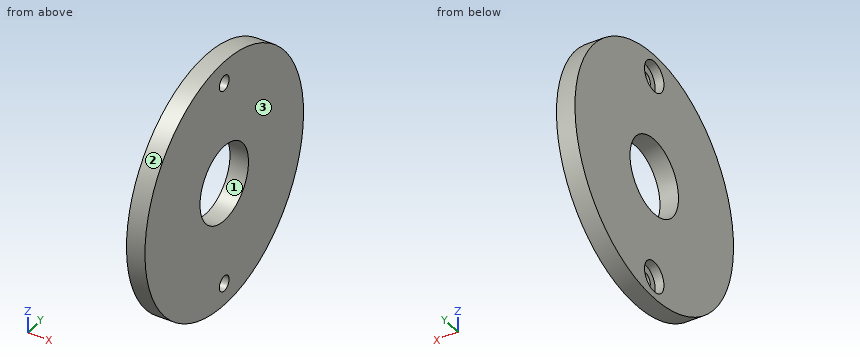
from build123d import *

# Parameters (mm, degrees)
F0_W     = 6.3
F0_H     = 29.5
F2_R     = 2.6
F3_DEPTH = 25
F4_R     = 5.2
F4_R_2   = 2.6
F5_DEPTH = 3


with BuildPart() as f1:
    # F0 (on Front) → F1 (revolve)
    with BuildSketch(Plane.XZ):
        with Locations((5.599999, 27.75)):
            Rectangle(F0_W, F0_H)
    revolve(axis=Axis((-4.686111, 0, 0), (-1, 0, 0)))

    # F2 (on face) → F3 (cut)
    with BuildSketch(Plane(origin=(2.449999, 0, 0), x_dir=(0, -1, 0), z_dir=(-1, 0, 0))):
        with Locations((0, 35)):
            Circle(F2_R)
        with Locations((0, -35)):
            Circle(F2_R)
    extrude(amount=-F3_DEPTH, mode=Mode.SUBTRACT)

    # F4 (on face) → F5 (cut)
    with BuildSketch(Plane(origin=(2.449999, 0, 0), x_dir=(0, -1, 0), z_dir=(-1, 0, 0))):
        with Locations((0, 35)):
            Circle(F4_R)
        with Locations((0, 35)):
            Circle(F4_R_2, mode=Mode.SUBTRACT)
        with Locations((0, -35)):
            Circle(F4_R)
        with Locations((0, -35)):
            Circle(F4_R_2, mode=Mode.SUBTRACT)
    extrude(amount=-F5_DEPTH, mode=Mode.SUBTRACT)


solid = f1.part
Can you work these out from the model? Positions are in its coordinate system, mm. Face numbers are marked on the shaded views. Give positions to 0.01 mm unless a question says otherwise; leave off trailing zeros. Loops run counter-clockwise (first coordinate to the right, second up) from the corner with the lowest first, then second, coordinate; pieces in that order, holes last. Notation, with made-up numbers: (86, -17) - (108, -17) arc R20 ccw to (108, 4) - close; hole circle Ø1 at (-4, -25.75). An arc over 180 degrees is marked (long way). Return JSON: item names as keys, results as strings.
1. I want a section at C-C on x = 3.5. Please give me the cut outline in (y, z).
Output values:
{"outline": "circle Ø85 at (0, 0); hole circle Ø26 at (0, 0); hole circle Ø10.4 at (0, -35); hole circle Ø10.4 at (0, 35)"}
2. We'd pull the mould along Z, two halves only. Please class the marked faces 1, 2 and 3: +Z half, -Z half, draft (parallel to the pull), parting line (faces both ways), or undercut.
Output values:
{"face 1": "undercut", "face 2": "parting line", "face 3": "draft"}
3. I want a section at D-D on z = -11. Please give me the cut outline in (x, y), and give its area (3 significant figures).
Output values:
{"outline": "(2.45, -41.05) - (8.75, -41.05) - (8.75, -6.93) - (2.45, -6.93) - close; (2.45, 6.93) - (8.75, 6.93) - (8.75, 41.05) - (2.45, 41.05) - close", "area": "430 mm²"}
4. If I drill on line 1 (Y direction, x = 7, z = 0); line 2 (Y direction, x = 6.5, z = -10.5); line 3 (X direction, y = -3, z = 31), over which ranges is the centre line in solid material (lowest first)?
Output values:
{"line 1": "y = -42.5 to -13, 13 to 42.5", "line 2": "y = -41.18 to -7.66, 7.66 to 41.18", "line 3": "x = 5.45 to 8.75"}
5. I want a section at A-A on z = 0. Please give me the cut outline in (x, y), and give its area (3 significant figures).
Output values:
{"outline": "(2.45, -42.5) - (8.75, -42.5) - (8.75, -13) - (2.45, -13) - close; (2.45, 13) - (8.75, 13) - (8.75, 42.5) - (2.45, 42.5) - close", "area": "372 mm²"}
6. I'm going to push flat-ended pins straight in: pin 1 Ø15.5 at (y, z) = (0, 0) entering from +X; pin 2 Ø4 at (y, z) = (-31.5, -30.5) entering from -X; pin 3 Ø2 at (x, y) = (4.5, 33.5) entering from -Z; pin 4 Ø3 at (y, z) = (2, 34) entering from -X. Where does each tip first touch, or does it pass through?
Output values:
{"pin 1": "passes through", "pin 2": "stops at x = 2.45", "pin 3": "stops at z = -27.39", "pin 4": "stops at x = 5.45"}
7. I want a section at B-B on y = 0. Please give me the cut outline in (x, z), and give its area (3 significant figures).
Output values:
{"outline": "(2.45, -42.5) - (8.75, -42.5) - (8.75, -37.6) - (5.45, -37.6) - (5.45, -40.2) - (2.45, -40.2) - close; (2.45, -29.8) - (5.45, -29.8) - (5.45, -32.4) - (8.75, -32.4) - (8.75, -13) - (2.45, -13) - close; (2.45, 13) - (8.75, 13) - (8.75, 32.4) - (5.45, 32.4) - (5.45, 29.8) - (2.45, 29.8) - close; (2.45, 40.2) - (5.45, 40.2) - (5.45, 37.6) - (8.75, 37.6) - (8.75, 42.5) - (2.45, 42.5) - close", "area": "275 mm²"}
